The model under review builds one solid part; all positions refer to its coordinate system, in mm. A direction names the side the tool comes from. Give positions to 0.01 mm unless a question says otherwise; leave off trailing zeros. Order: outer loops, then holes, each group sorted by start corner. A loop starts at its lowest first (then second) coordinate and runs counter-clockwise, first axis right, second up. Notation, with made-up numbers: (56.5, -5.75) - (87.5, -5.75) arc R23 ccw to (87.5, 29.25) - close; hole circle Ø8 at (2.5, -14). An arc over 180 degrees is marked (long way). Use a Markdown table: item, result. Add a question column.
Autodesk Inventor part; units mm, degrees
ref_plane "YZ Plane" through (0, 0, 0) normal (1, 0, 0) x (0, 1, 0)
ref_plane "XZ Plane" through (0, 0, 0) normal (0, 1, 0) x (-1, 0, 0)
ref_plane "XY Plane" through (0, 0, 0) normal (0, 0, 1) x (1, 0, 0)
sketch "スケッチ1" plane through (0, 0, 0) normal (0, 0, 1) x (1, 0, 0)
  circle A0 centre (0, 0) radius 10.5 construction
  circle A1 centre (-13.5, 1) radius 1.35
  line L0 (-13.5, 28) -> (13.5, 28) construction
  line L1 (13.5, 28) -> (13.5, 1) construction
  line L2 (13.5, 1) -> (-13.5, 1) construction
  line L3 (-13.5, 1) -> (-13.5, 28) construction
  circle A2 centre (-13.5, 28) radius 1.35
  circle A3 centre (13.5, 1) radius 1.35
  circle A4 centre (13.5, 28) radius 1.35
  line L4 (-19.75, 10) -> (-19.75, 7.1)
  line L5 (-19.75, 10) -> (19.75, 10)
  line L6 (19.75, 10) -> (19.75, 7.1)
  line L7 (-19.75, -7.1) -> (-19.75, -10)
  line L8 (-19.75, -10) -> (19.75, -10)
  line L9 (19.75, -7.1) -> (19.75, -10)
  line L10 (-19.75, 5) -> (-21.75, 5)
  line L11 (-21.75, 5) -> (-21.75, -5)
  line L12 (-21.75, -5) -> (-19.75, -5)
  arc A5 (-19.75, 5) -> (-19.75, 7.1) centre (-19.75, 6.05) ccw
  arc A6 (-19.75, -7.1) -> (-19.75, -5) centre (-19.75, -6.05) ccw
  line L13 (19.75, 5) -> (21.75, 5)
  line L14 (21.75, 5) -> (21.75, -5)
  line L15 (21.75, -5) -> (19.75, -5)
  arc A7 (19.75, 7.1) -> (19.75, 5) centre (19.75, 6.05) ccw
  line L16 (0, 28) -> (0, 0) construction
  arc A8 (19.75, -5) -> (19.75, -7.1) centre (19.75, -6.05) ccw
  line L17 (-21.75, 0) -> (21.75, 0) construction
  circle A9 centre (0, 0) radius 6.05
  point P0 (0, 10)
  dimension "d8" = 21
  dimension "d10" = 27
  dimension "d12" = 1
  dimension "d13" = 2.7
  dimension "d38" = 27
  dimension "d44" = 27
  dimension "d47" = 1.05
  dimension "d48" = 39.5
  dimension "d49" = 2
  dimension "d50" = 10
  dimension "d51" = 5
  dimension "d52" = 12.1
extrude "押し出し1" add sketch "スケッチ1" along normal blind 2 contours L5 L6 A7 L13 L14 L15 A8 L9 L8 L7 A6 L12 L11 L10 A5 L4
sketch "スケッチ2" plane through (0, 0, 2) normal (0, 0, 1) x (1, 0, 0)
  circle A0 centre (0, 0) radius 6.05
  circle A1 centre (-13.5, 1) radius 1.35
  line L0 (-19.75, -10) -> (19.75, -10)
  line L1 (19.75, 10) -> (-19.75, 10)
  line L2 (-11.8485, 3) -> (-7.4162, 3)
  arc A2 (7.4162, 3) -> (-7.4162, 3) centre (0, 0) ccw
  line L3 (7.4162, 3) -> (11.8485, 3)
  line L4 (-18.4641, 12.448) -> (18.4641, 12.448)
  line L5 (-18.4641, 12.448) -> (-11.8485, 3)
  line L6 (11.8485, 3) -> (18.4641, 12.448)
  line L7 (-11.8485, -3) -> (-7.4162, -3)
  line L8 (-11.8485, -3) -> (-24.333, -20.8295)
  line L9 (-24.333, -20.8295) -> (24.333, -20.8295)
  line L10 (11.8485, -3) -> (7.4162, -3)
  line L11 (11.8485, -3) -> (24.333, -20.8295)
  arc A3 (-7.4162, -3) -> (7.4162, -3) centre (0, 0) ccw
  line L12 (-21.75, 5) -> (-21.75, -5)
  line L13 (-16.75, 10) -> (-19.75, 10) construction
  line L14 (0, 0) -> (-21.75, 0) construction
  line L15 (-19.75, -10) -> (-16.75, -10) construction
  line L16 (-19.75, -10) -> (19.75, -10) construction
  line L17 (0, 0) -> (0, 10) construction
  line L18 (19.75, 10) -> (16.75, 10) construction
  line L19 (19.75, -10) -> (16.75, -10) construction
  circle A4 centre (-13.5, 1) radius 2.5 construction
  dimension "d57" = 8
  dimension "d58" = 3
  dimension "d60" = 6
  dimension "d64" = 3
  dimension "d65" = 5
extrude "押し出し2" cut sketch "スケッチ2" against normal blind 10 contours L8 L7 A3 L10 L11 L0 | L0 L11 L9 L8 | L6 L3 A2 L2 L5 L1 | L1 L5 L4 L6
fillet "フィレット1" radius 2 11 edges at (-11.8485, 3, 1) (-7.4162, 3, 1) (7.4162, 3, 1) (11.8485, -3, 1) (7.4162, -3, 1) (-7.4162, -3, 1) (-11.8485, -3, 1) (-16.75, -10, 1) (-16.75, 10, 1) (16.75, 10, 1) (16.75, -10, 1)
equation "\"d38\" = d10"
equation "\"d44\" = d10"
equation "\"d50\" = d11"
equation "\"d51\" = d28"
equation "\"d60\" = 2 * d58"
properties part number "足首_サブフレーム_1_2" material "アルミニウム 2014-T4"
Q1. Machinability: for faces 1 (the flat face through (-19.75, 9, 1)), 2 (the cylindrical face through (-7.673, -3.261, 0.986)), 3 (the cylindrical face through (16.86, 9.77, 0.99)), 4 (the flat face through (-21, -5, 1)), which of the approach directions +Z, -Z, +X, -X, +Y, -Y give a long, thin tool a straight path to every point of the face, cutting with its end or side? Answer none if there is none.
Q2. We need section A-A (x = 5). Write out the cut boundary in (y, z) (3 decimals), plus the area to 3 significant figures.
Q3. We need section C-C (y = 0.5). Write out the cut boundary in (x, z).
Q4. Wall thickness on probe 1 along X at (y, z) = (4.5, 1.2); probe 2 along Y at (x, z) = (-13.5, 0.5); probe 3 along Y at (x, z) = (-3.5, 1.2): over which ranges is each line inside the solid? List them lowest first.
Q5. Clearance check with flat-ended pins moving along their axes: P1, Ø0.6, axis at y = 9, z = 1, coming from the +X side; P2, Ø1, axis at x = -20.5, z = 1, coming from the +Y side; P3, Ø1, axis at y = -9, z = 1.5, coming from the -X side; P4, Ø9.5, axis at x = 0, y = 0, coming from the -Z side (3 decimals). State where each tip first meets the part, or that it passes through.
Q6. We need section D-D (z = 1.55). Count the separate pieces of the cut face and the enclosed holes in it, plus the area to 3 significant figures.
Q7. Draft analysis for pull direction X (two halves, no side actions). For faces 5 (the cylindrical face through (12.15, 0.94, 0.99)), 6 (the flat face through (19.75, -9, 1)), 7 (the flat face through (-21.75, 0, 1)), state which applies: pulls with the +X half, pulls with the -X half, needs draft (parallel to the pull), parting line crosses it, or undercut.
Q8. We need section B-B (y = 7.5). Write out the cut boundary in (x, z), plus the area to 3 significant figures.
Here are the results:
| question | item | result |
|---|---|---|
| 1 | face 1 | +Z, -Z, -X, +Y |
| 1 | face 2 | +Z, -Z, -Y |
| 1 | face 3 | +Z, -Z, +Y |
| 1 | face 4 | +Z, -Z, -X, -Y |
| 2 | outline | (-6.245, 0) - (-3.406, 0) - (-3.406, 2) - (-6.245, 2) - close; (3.406, 0) - (6.245, 0) - (6.245, 2) - (3.406, 2) - close |
| 2 | area | 11.4 mm2 |
| 3 | outline | (-21.75, 0) - (-14.75, 0) - (-14.75, 2) - (-21.75, 2) - close; (-12.25, 0) - (-6.03, 0) - (-6.03, 2) - (-12.25, 2) - close; (6.03, 0) - (12.25, 0) - (12.25, 2) - (6.03, 2) - close; (14.75, 0) - (21.75, 0) - (21.75, 2) - (14.75, 2) - close |
| 4 | probe 1 | -21.75 to -12.9, -6.61 to -4.04, 4.04 to 6.61, 12.9 to 21.75 |
| 4 | probe 2 | -5.36 to -0.35, 2.35 to 5.36 |
| 4 | probe 3 | -7.19 to -4.93, 4.93 to 7.19 |
| 5 | P1 | x = 19.75 |
| 5 | P2 | y = 5 |
| 5 | P3 | x = -19.75 |
| 5 | P4 | through |
| 6 | separate pieces | 1 |
| 6 | enclosed holes | 3 |
| 6 | area | 404 mm2 |
| 7 | face 5 | undercut |
| 7 | face 6 | pulls with the +X half |
| 7 | face 7 | pulls with the -X half |
| 8 | outline | (-19.75, 0) - (-15, 0) - (-15, 2) - (-19.75, 2) - close; (-2.78, 0) - (2.78, 0) - (2.78, 2) - (-2.78, 2) - close; (15, 0) - (19.75, 0) - (19.75, 2) - (15, 2) - close |
| 8 | area | 30.1 mm2 |
